Study the drawing (mm; zero at the part's minimum x, y, z) and answer. Coordinates: 2 decimals unless noted, no trailing zeros. Loops run counter-clockwise (first coordinate to the right, second up) from the corner with the lowest first, then second, coordinate; pieces in that order, holes last. Notation, with made-up numbers: (-33.75, -29.5) -> (1.25, -29.5) arc R12 ccw to (1.25, -7.5) -> close; hole circle Ø3 at (42, -38). An arc over 180 degrees is marked (long way). One line per question, with ' | ' between items.
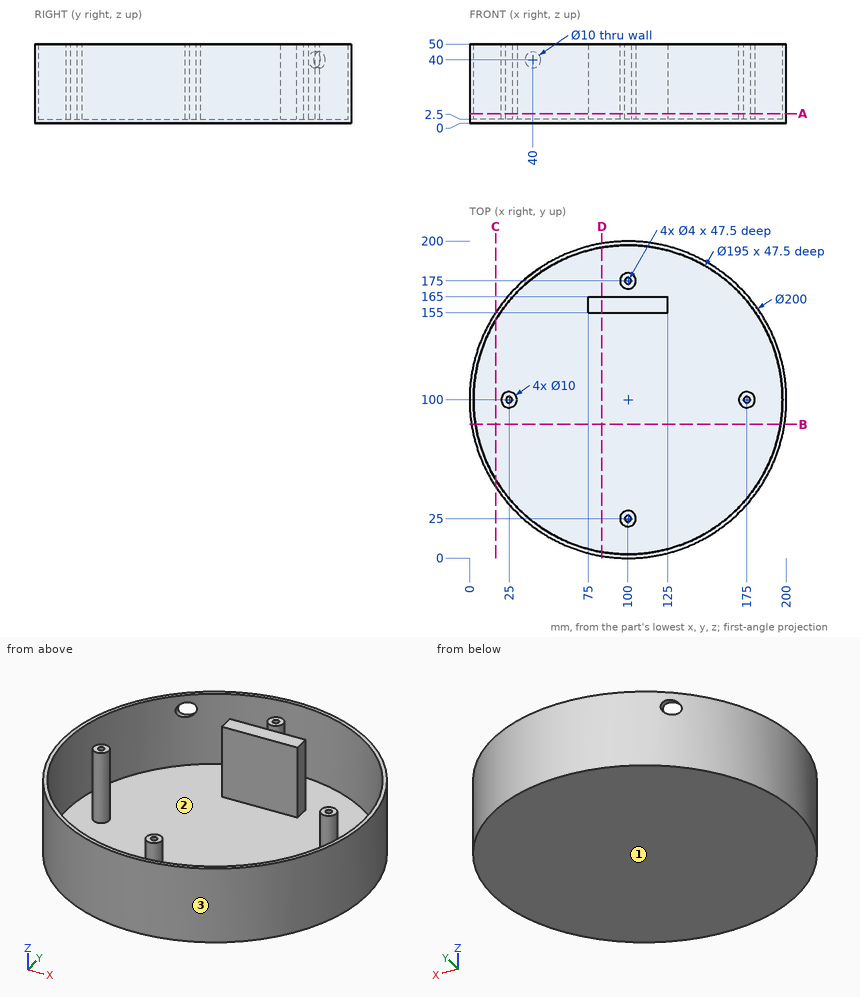
1) The mould has two halves that part along Y. Classify the marked faces 1, 2 and 3: released by +Y, released by -Y, zero draft, split by the parting line, or undercut.
Check values:
face 1: zero draft | face 2: undercut | face 3: split by the parting line
2) Find section D-D (x = 83.5). Write down the section's boundary in (y, z), plus the area to 3 significant figures.
Check values:
outline: (1.37, 0) -> (198.63, 0) -> (198.63, 50) -> (196.09, 50) -> (196.09, 2.5) -> (165, 2.5) -> (165, 50) -> (155, 50) -> (155, 2.5) -> (3.91, 2.5) -> (3.91, 50) -> (1.37, 50) -> close | area: 1,210 mm^2
3) Find section A-A (z = 6). State how many separate pieces and enclosed holes the cut face has, plus the area to 3 significant figures.
Check values:
separate pieces: 6 | enclosed holes: 5 | area: 2,320 mm^2
4) Find the intervals of material crossed by line 1 along X through (y, z) = (179.5, 19.5); line 2 along Y through (x, z) = (103.5, 34.5); line 3 along X through (y, z) = (173.5, 24), in increasing order.
Check values:
line 1: x = 39.34 to 43.56, 97.82 to 102.18, 156.44 to 160.66 | line 2: y = 0.06 to 2.56, 21.43 to 28.57, 155 to 165, 171.43 to 178.57, 197.44 to 199.94 | line 3: x = 32.19 to 35.94, 95.23 to 98.68, 101.32 to 104.77, 164.06 to 167.81
5) Find section B-B (y = 84.5). Write down the section's boundary in (x, z), plus the area to 3 significant figures.
Check values:
outline: (1.21, 0) -> (198.79, 0) -> (198.79, 50) -> (196.26, 50) -> (196.26, 2.5) -> (3.74, 2.5) -> (3.74, 50) -> (1.21, 50) -> close | area: 734 mm^2
6) Flat-ended cylindrical pins translate along their axes: pin 1 (8 mm diameter, centred on x = 41, z = 39, fed in from -Y); pin 2 (1.5 mm diameter, centred on y = 33.5, z = 8, fed in from +X); pin 3 (10 mm diameter, centred on y = 58, z = 38, fed in from +X); pin 4 (2 mm diameter, centred on x = 99, y = 175.5, fed in from +Z). Find the tip coordinate at first contact, or state that the pin passes through.
Check values:
pin 1: stops at y = 16.48 | pin 2: stops at x = 175.35 | pin 3: stops at x = 192.9 | pin 4: stops at z = 50
7) Find section C-C (x = 16.5). Write down the section's boundary in (y, z) (3 decimals).
Check values:
outline: (44.975, 0) -> (155.025, 0) -> (155.025, 50) -> (150.339, 50) -> (150.339, 2.5) -> (49.661, 2.5) -> (49.661, 50) -> (44.975, 50) -> close
